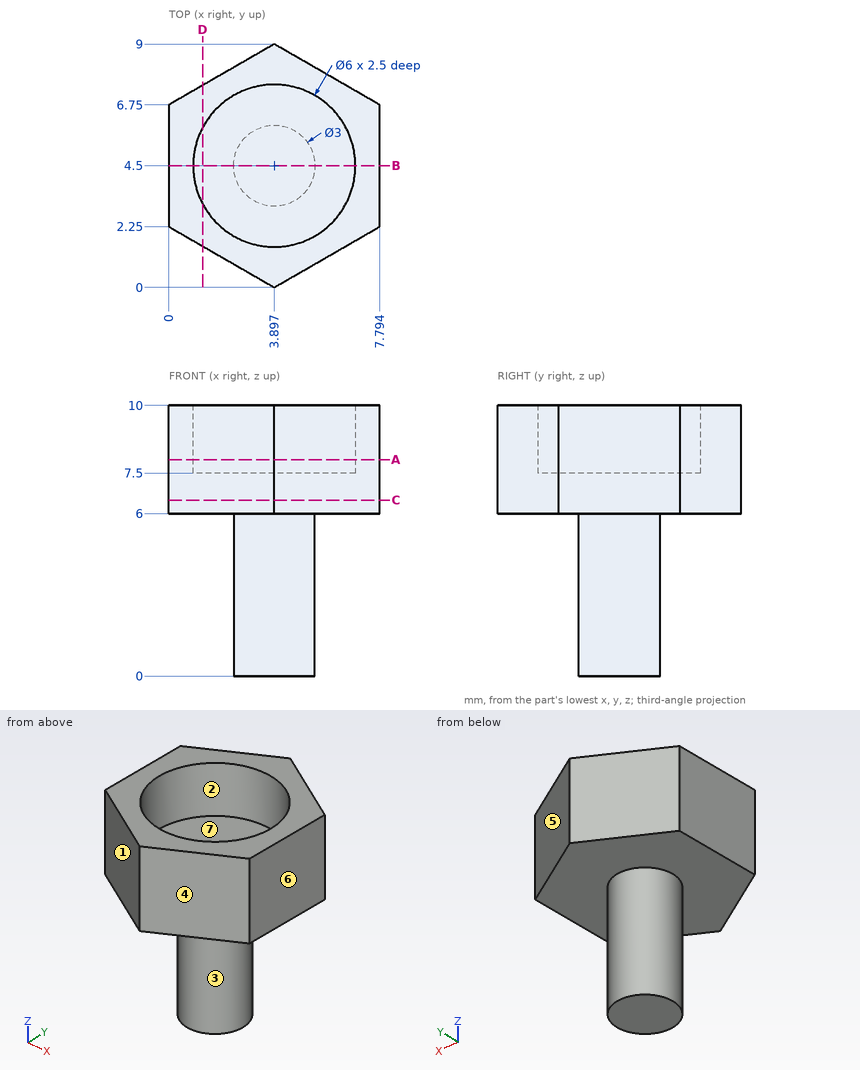
Input: dimensioned drawing with shaded views. Units: mm. Origin: part minimum x, y, z. A direction names the side the tool comes from. Coordinates: 2 decimals unless noted, no trailing zeros. Order: outer loops, then holes, each group sorted by start corner. A loop starts at its lowest first (then second) coordinate and runs counter-clockwise, first axis right, second up. Notation, with made-up numbers: (7, 52) -> (59, 52) arc R32 ccw to (59, 78) -> close; hole circle Ø4 at (70.5, -23). An arc over 180 degrees is marked (long way). Use CSV: the item, a comma, the result in double quotes.
1) Section A-A on z = 8. Output: boundary loops of the cut face in (x, y).
Findings:
outline,"(0, 2.25) -> (3.9, 0) -> (7.79, 2.25) -> (7.79, 6.75) -> (3.9, 9) -> (0, 6.75) -> close; hole circle Ø6 at (3.9, 4.5)"
2) Access query for the marked faces 1, 2 and 3. Directions: +Z, -Z, +X, -X, +Y, -Y. A direction counts if a zero-diameter tool reaches every point of the face in a straight line with its end or side. Return the directions, or none.
Findings:
face 1,"+Z, -Z, -X, -Y"
face 2,"+Z"
face 3,"-Z"
3) Line query: line 1 (Z direction, x = 0.75, y = 5.5); line 2 (Z direction, x = 6, y = 6.5); line 3 (X direction, y = 2.5, z = 9.25) (1 decimal). Output: solid intervals per line, ascending.
Findings:
line 1,"z = 6 to 10"
line 2,"z = 6 to 7.5"
line 3,"x = 0 to 1.7, 6.1 to 7.8"
4) Mould query, pull axis Y, two halves, no side actions, for the marked faces 4, 5, 6 and 7. Classes: +Y half, -Y half, draft (parallel to the pull), parting line (faces both ways), or undercut.
Findings:
face 4,"-Y half"
face 5,"+Y half"
face 6,"draft"
face 7,"undercut"
5) Section C-C on z = 6.5. Output: boundary loops of the cut face in (x, y), then the cut area to 3 significant figures.
Findings:
outline,"(0, 2.25) -> (3.9, 0) -> (7.79, 2.25) -> (7.79, 6.75) -> (3.9, 9) -> (0, 6.75) -> close"
area,"52.6 mm^2"
6) Pin query (flat end, axial travel): pin 1 Ø4 at (x, z) = (3.5, 6.5) entering from -Y; pin 2 Ø1 at (y, z) = (7.5, 5) entering from +X. Return the tip coordinate at first contact, or that it passes through.
Findings:
pin 1,"stops at y = 0"
pin 2,"passes through"
7) Section D-D on x = 1.25. Output: boundary loops of the cut face in (y, z), then the cut area to 3 significant figures.
Findings:
outline,"(1.53, 6) -> (7.47, 6) -> (7.47, 10) -> (5.91, 10) -> (5.91, 7.5) -> (3.09, 7.5) -> (3.09, 10) -> (1.53, 10) -> close"
area,"16.7 mm^2"
8) Section B-B on y = 4.5. Output: boundary loops of the cut face in (x, z), then the cut area to 3 significant figures.
Findings:
outline,"(0, 6) -> (2.4, 6) -> (2.4, 0) -> (5.4, 0) -> (5.4, 6) -> (7.79, 6) -> (7.79, 10) -> (6.9, 10) -> (6.9, 7.5) -> (0.9, 7.5) -> (0.9, 10) -> (0, 10) -> close"
area,"34.2 mm^2"
